Part model, mm, in its own coordinate system. Face numbers are marked on the shaded views. A direction names the side the tool comes from. Give positions to 0.01 mm unless a question says otherwise; leave off trailing zeros. Write each loop counter-clockwise with the first axis right and the second up, starting at its lowest first coordinate (ties: lowest second). Pieces come first, ordered by that corner, then holes.
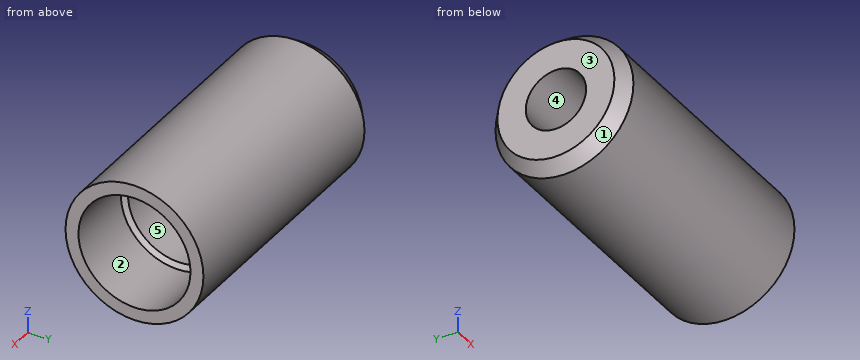
from build123d import *

# Parameters (mm, degrees)
F_7_8_14_TAPPED_HOLE1_D     = 20.6375
F_7_8_14_TAPPED_HOLE1_DEPTH = 12.7
F_7_8_14_TAPPED_HOLE1_TIP   = 6.200130513


with BuildPart() as part:
    # Sketch2 → Revolve1 (revolve)
    with BuildSketch(Plane.XY, mode=Mode.PRIVATE) as revolve1_sk:
        Polygon((0, 10.771663062), (2.558989547, 12.7), (50.8, 12.7), (50.8, 9.35355), (25.4, 9.35355), (25.4, 5.55625), (0, 5.55625), align=None)
    revolve(revolve1_sk.sketch.rotate(Axis((0, 0, 0), (1, 0, 0)), 90), axis=Axis((0, 0, 0), (1, 0, 0)))

    # 7/8-14 Tapped Hole1
    with Locations(Plane(origin=(50.8, 0, 0), x_dir=(0, 0, -1), z_dir=(1, 0, 0))):
        with Locations((0, 0)):
            Hole(F_7_8_14_TAPPED_HOLE1_D / 2, depth=F_7_8_14_TAPPED_HOLE1_DEPTH)
            with Locations((0, 0, -(F_7_8_14_TAPPED_HOLE1_DEPTH + F_7_8_14_TAPPED_HOLE1_TIP / 2))):  # 118° drill point
                Cone(0, F_7_8_14_TAPPED_HOLE1_D / 2, F_7_8_14_TAPPED_HOLE1_TIP, mode=Mode.SUBTRACT)


solid = part.part
1) Saw through at C-C (x = 10.5). Write the cut outline in (y, z).
Check result:
outline: circle Ø25.4 at (0, 0); hole circle Ø11.11 at (0, 0)
2) 3-axis set-ups, long thin cutter, end or side, ignore diameter. For the marked faces 4 and 5: which of +Z, -Z, +X, -X, +Y, -Y reach the whole face in a straight line?
Check result:
face 4: +X, -X
face 5: +X
3) Saw through at A-A (y = 0). Write the cut outline in (x, z).
Check result:
outline: (0, -10.77) - (2.56, -12.7) - (50.8, -12.7) - (50.8, -10.32) - (38.1, -10.32) - (37.52, -9.35) - (25.4, -9.35) - (25.4, -5.56) - (0, -5.56) - close; (0, 5.56) - (25.4, 5.56) - (25.4, 9.35) - (37.52, 9.35) - (38.1, 10.32) - (50.8, 10.32) - (50.8, 12.7) - (2.56, 12.7) - (0, 10.77) - close
4) Drill centre lines: L1, parallel to Y at x = 33.75, z = 0; L2, parallel to Y at x = 47.5, z = 0; L3, parallel to X at y = 6, z = 5.75. Where is each one in solid material? Low to high.
Check result:
L1: y = -12.7 to -9.35, 9.35 to 12.7
L2: y = -12.7 to -10.32, 10.32 to 12.7
L3: x = 0 to 25.4
5) Flat gauge pins, fed straight in: P1, Ø14.5, axis at y = 0, z = 0, coming from the +X side; P2, Ø1.5, axis at x = 9.5, z = 1, coming from the +Y side; P3, Ø1, axis at x = 36.5, y = 5, coming from the +Z side. Where does each tip first touch, or does it go through?
Check result:
P1: stops at x = 25.4
P2: stops at y = 12.7
P3: stops at z = 11.88
6) Mould opens along Y. For the marked faces 1, 2 and 3 say: +Y half, -Y half, draft (parallel to the pull), parting line (faces both ways), or undercut.
Check result:
face 1: parting line
face 2: undercut
face 3: draft
